Read the model definition and answer for the solid it produces. Units are mm, in the model's axes. A direction names the side the tool comes from. Give positions to 0.01 mm unless a question says otherwise; leave off trailing zeros. Order: outer loops, then holes, each group sorted by start corner. A loop starts at its lowest first (then second) coordinate and runs counter-clockwise, first axis right, second up. Notation, with made-up numbers: (71.25, 25.5) -> (89.25, 25.5) arc R26 ccw to (89.25, 53.5) -> close; hole circle Ø4 at (23, 77). An arc over 180 degrees is marked (long way). Answer as CSV lines item,"result". Start each with the question number.
1) Find section B-B (z = -1.5). Determine the outline of the cut face in (x, y).
2) For faces 1 (the face through (-21.404, 2.498, 49.3)), 2 (the face through (-21.085, 3.983, -4.93)), 3 (the face through (-18.3, 2.93, 104.93)), determine the directions among +Z, -Z, +X, -X, +Y, -Y from which every point of the face is accessible in a straight line to the end or side of a thin tool.
3) Straight lines are drawn through the part: L1, parallel to Z at x = -19.95, y = 5.1; L2, parallel to Y at x = -19.7, z = 77; L3, parallel to Y at x = -20.85, z = 19. For each, find the intervals that lie inside material, in ascending order. Write a range as from..to.
4) Find section A-A (z = 85). Determine the outline of the cut face in (x, y), and give its area (3 significant figures).
```python
from build123d import *

# Parameters (mm, degrees)
BOSS_EXTRUDE1_DEPTH = 100
SKETCH3_R           = 1.5
BOSS_EXTRUDE2_DEPTH = 10
SKETCH4_R           = 1.5
BOSS_EXTRUDE3_DEPTH = 10


with BuildPart() as part:
    # Sketch2 → Boss-Extrude1 (new body)
    with BuildSketch(Plane.XY):
        Polygon((-18.575897145, 5.546778343), (-20.884739637, 5.495987805), (-21.995174987, 3.471076285), (-20.796767845, 1.496955302), (-18.487925352, 1.54774584), (-17.377490002, 3.57265736), align=None)
    extrude(amount=BOSS_EXTRUDE1_DEPTH)

    # Sketch3 → Boss-Extrude2 (add)
    with BuildSketch(Plane.XY.offset(100)):
        with Locations((-19.683896115, 3.505839662)):
            Circle(SKETCH3_R)
    extrude(amount=BOSS_EXTRUDE2_DEPTH)

    # Sketch4 → Boss-Extrude3 (add)
    with BuildSketch(Plane(origin=(0, 0, 0), x_dir=(-1, 0, 0), z_dir=(0, 0, -1))):
        with Locations((19.653785762, 3.532451742)):
            Circle(SKETCH4_R)
    extrude(amount=BOSS_EXTRUDE3_DEPTH)


solid = part.part
```
Findings below:
1,outline,"circle Ø3 at (-19.65, 3.53)"
2,face 1,"+Z, -Z, -X, -Y"
2,face 2,"-Z"
2,face 3,"+Z"
3,L1,"0..100"
3,L2,"1.52..5.52"
3,L3,"1.58..5.5"
4,outline,"(-22, 3.47) -> (-20.8, 1.5) -> (-18.49, 1.55) -> (-17.38, 3.57) -> (-18.58, 5.55) -> (-20.88, 5.5) -> close"
4,area,"13.9 mm²"
